Geometry check sheet. Reference: the model listing, model coordinates, mm. Give positions to 0.01 mm unless a question says otherwise; leave off trailing zeros. Loops run counter-clockwise (first coordinate to the right, second up) from the corner with the lowest first, then second, coordinate; pieces in that order, holes last. Notation, with made-up numbers: (47, 41) - (78, 41) arc R20 cw to (78, 72) - close; hole circle Ø11 at (48, 9). An arc over 180 degrees is marked (long way). Use a Markdown table: item, result. Add a question column.
1. Material ranges on L1, parallel to X at y = 2, z = 40; L2, parallel to Y at x = -25, z = -62; L3, parallel to X at y = 37.5, z = 17, recorded low to high.
2. Cross-section at B-B on z = 40. Enter the section's corners in (x, y).
3. Cross-section at D-D on z = 1.5. Enter the section's corners in (x, y), and give its area (3 significant figures).
4. Depth check by flat-ended pin: P1, Ø0.6, axis at x = 44, y = 2, coming from the -Z side; P2, Ø4, axis at y = 13.5, z = 47.5, coming from the -X side; P3, Ø1.6, axis at x = -46.5, y = 2, coming from the +Z side; P4, Ø4.5, axis at x = -45, z = 40, coming from the +Y side. Enter the tip coordinate at first touch or a pass-through.
5. Cross-section at A-A on x = 45. Enter the section's corners in (y, z), and give its area (3 significant figures).
6. Cross-section at C-C on y = 23.25. Enter the section's corners in (x, z).
from build123d import *

# Parameters (mm, degrees)
SKETCH_1_W          = 77
SKETCH_1_H          = 129
EXTRUDE_1_DEPTH     = 46.5
SKETCH_2_W          = 12.5
SKETCH_2_H          = 13
SKETCH_2_R          = 2.6
EXTRUDE_2_DEPTH     = 3
SKETCH_3_R          = 4
CUT_EXTRUDE_1_DEPTH = 5
FILLET_1_R          = 1


with BuildPart() as part:
    # 草图1 → 凸台-拉伸1 (new body)
    with BuildSketch(Plane(origin=(0, 0, 0), x_dir=(1, 0, 0), z_dir=(0, 1, 0))):
        Rectangle(SKETCH_1_W, SKETCH_1_H)
    extrude(amount=EXTRUDE_1_DEPTH)

    # 草图2 → 凸台-拉伸2 (add)
    # profile 1 of 4: a face of its own
    with BuildSketch(Plane.XZ):
        with Locations((-44.75, 39.75)):
            Rectangle(SKETCH_2_W, SKETCH_2_H)
        with Locations(Location((-45, 40, 0), (0, 0, 270))):
            Circle(SKETCH_2_R, mode=Mode.SUBTRACT)
    # profile 2 of 4: a face of its own
    with BuildSketch(Plane.XZ):
        with Locations((44.75, 39.75)):
            Rectangle(SKETCH_2_W, SKETCH_2_H)
        with Locations(Location((45, 40, 0), (0, 0, 90))):
            Circle(SKETCH_2_R, mode=Mode.SUBTRACT)
    # profile 3 of 4: a face of its own
    with BuildSketch(Plane.XZ):
        with Locations((44.75, -39.75)):
            Rectangle(SKETCH_2_W, SKETCH_2_H)
        with Locations(Location((45, -40, 0), (0, 0, 270))):
            Circle(SKETCH_2_R, mode=Mode.SUBTRACT)
    # profile 4 of 4: a face of its own
    with BuildSketch(Plane.XZ):
        with Locations((-44.75, -39.75)):
            Rectangle(SKETCH_2_W, SKETCH_2_H)
        with Locations(Location((-45, -40, 0), (0, 0, 90))):
            Circle(SKETCH_2_R, mode=Mode.SUBTRACT)
    extrude(amount=-EXTRUDE_2_DEPTH)

    # 草图3 → 切除-拉伸1 (cut)
    with BuildSketch(Plane(origin=(0, 0, -64.5), x_dir=(-1, 0, 0), z_dir=(0, 0, -1))):
        with Locations((25, 23.25)):
            Circle(SKETCH_3_R)
    extrude(amount=-CUT_EXTRUDE_1_DEPTH, mode=Mode.SUBTRACT)

    # 圆角1
    fillet_1_edges = [part.edges().sort_by_distance(p)[0] for p in [
        (-38.5, 46.5, 0),
        (-38.5, 0, 55.375),
        (0, 46.5, 64.5),
        (-44.75, 0, 46.25),
        (-51, 0, 39.75),
        (-44.75, 0, 33.25),
        (-45, 0, 42.6),
        (38.5, 0, 0),
        (44.75, 0, 33.25),
        (51, 0, 39.75),
        (44.75, 0, 46.25),
        (45, 0, 37.4),
        (38.5, 0, -55.375),
        (44.75, 0, -46.25),
        (51, 0, -39.75),
        (44.75, 0, -33.25),
        (45, 0, -37.4),
        (38.5, 46.5, 0),
        (0, 0, 64.5),
        (-38.5, 0, 0),
        (-38.5, 0, -55.375),
        (-44.75, 0, -33.25),
        (-51, 0, -39.75),
        (-44.75, 0, -46.25),
        (-45, 0, -42.6),
        (0, 0, -64.5),
        (38.5, 0, 55.375),
        (0, 46.5, -64.5),
    ]]
    fillet(fillet_1_edges, radius=FILLET_1_R)


solid = part.part
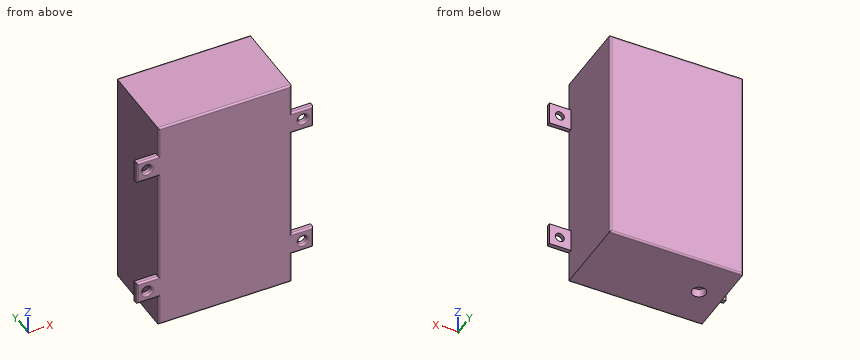
Values found:
| question | item | result |
|---|---|---|
| 1 | L1 | x = -51 to -47.6, -42.4 to 42.4, 47.6 to 51 |
| 1 | L2 | y = 0 to 19.25, 27.25 to 46.5 |
| 1 | L3 | x = -38.5 to 38.5 |
| 2 | outline | (-51, 1) arc R1 ccw to (-50, 0) - (-48.6, 0) arc R1 ccw to (-47.6, 1) - (-47.6, 3) - (-51, 3) - close; (-42.4, 1) arc R1 ccw to (-41.4, 0) - (41.4, 0) arc R1 ccw to (42.4, 1) - (42.4, 3) - (38.5, 3) - (38.5, 45.5) arc R1 ccw to (37.5, 46.5) - (-37.5, 46.5) arc R1 ccw to (-38.5, 45.5) - (-38.5, 3) - (-42.4, 3) - close; (47.6, 1) arc R1 ccw to (48.6, 0) - (50, 0) arc R1 ccw to (51, 1) - (51, 3) - (47.6, 3) - close |
| 3 | outline | (-38.5, 1) arc R1 ccw to (-37.5, 0) - (37.5, 0) arc R1 ccw to (38.5, 1) - (38.5, 45.5) arc R1 ccw to (37.5, 46.5) - (-37.5, 46.5) arc R1 ccw to (-38.5, 45.5) - close |
| 3 | area | 3,580 mm2 |
| 4 | P1 | stops at z = -46.25 |
| 4 | P2 | stops at x = -38.5 |
| 4 | P3 | stops at z = 46.25 |
| 4 | P4 | passes through |
| 5 | outline | (0, -45.25) arc R1 ccw to (1, -46.25) - (3, -46.25) - (3, -42.6) - (1, -42.6) arc R1 ccw to (0, -43.6) - close; (0, -36.4) arc R1 ccw to (1, -37.4) - (3, -37.4) - (3, -33.25) - (1, -33.25) arc R1 ccw to (0, -34.25) - close; (0, 34.25) arc R1 ccw to (1, 33.25) - (3, 33.25) - (3, 37.4) - (1, 37.4) arc R1 ccw to (0, 36.4) - close; (0, 43.6) arc R1 ccw to (1, 42.6) - (3, 42.6) - (3, 46.25) - (1, 46.25) arc R1 ccw to (0, 45.25) - close |
| 5 | area | 45.1 mm2 |
| 6 | outline | (-38.5, -64.5) - (-29, -64.5) - (-29, -59.5) - (-21, -59.5) - (-21, -64.5) - (38.5, -64.5) - (38.5, 64.5) - (-38.5, 64.5) - close |
